Source: CAD feature listing. Evaluate the final solid. Frame: model axes, mm. A direction names the side the tool comes from. Give positions to 0.01 mm unless a question says otherwise; leave off trailing zeros. Loops run counter-clockwise (first coordinate to the right, second up) from the corner with the lowest first, then second, coordinate; pieces in that order, holes last. Notation, with made-up numbers: (-1.75, -39) -> (14.25, -39) arc R24 cw to (14.25, -26) -> close; hole circle Ø10 at (86.25, 67.25). An arc over 180 degrees is marked (long way). Return JSON: item names as keys, results as strings. Group by question number.
(1) Pin query (flat end, axial travel): pin 1 (1.5 mm diameter, centred on x = 1020.5, y = -41.5, fed in from -Z). Return the tip coordinate at first contact, or that it passes through.
(2) Cut plane B-B on y = 353. Return loops of the section in (x, z), then the cut area to 3 significant figures.
(3) Ray query, line 1 (Z direction, x = 579, y = 403.5). Return the intervals inside material, ascending. Write a range as from..to.
(4) Cut plane A-A on x = 301.5. Return loops of the section in (y, z) (3 decimals).
(5) Access query for faces 1 (the face through (1372.587, 32, 101)), 2 (the face through (445, -163, 0)), 3 (the face through (445, 297, 0)). Directions: +Z, -Z, +X, -X, +Y, -Y. A direction counts if a zero-diameter tool reaches every point of the face in a straight line with its end or side. Return the directions, or none.
```python
from build123d import *

# Parameters (mm, degrees)
F0_W     = 1828.8
F0_H     = 914.4
F1_DEPTH = 203.2
F3_R     = 3.175
F4_DEPTH = 1828.8


with BuildPart() as f1:
    # F0 (on Top) → F1 (new body)
    with BuildSketch(Plane.XY):
        with Locations((458.187128, 38.50697)):
            Rectangle(F0_W, F0_H)
    extrude(amount=F1_DEPTH)

    # F3 (on face) → F4 (join)
    with BuildSketch(Plane.YZ.offset(1372.587128)):
        with Locations((89.30697, 0)):
            Circle(F3_R)
    extrude(amount=-F4_DEPTH)


solid = f1.part
```
Answers:
{
 "1": {"pin 1": "z = 0"},
 "2": {"outline": "(-456.21, 0) -> (1372.59, 0) -> (1372.59, 203.2) -> (-456.21, 203.2) -> close", "area": "372,000 mm²"},
 "3": {"line 1": "0..203.2"},
 "4": {"outline": "(-418.693, 0) -> (86.132, 0) arc R3.175 ccw to (92.482, 0) -> (495.707, 0) -> (495.707, 203.2) -> (-418.693, 203.2) -> close"},
 "5": {"face 1": "+Z, -Z, +X, +Y, -Y", "face 2": "-Z, +X, -X, -Y", "face 3": "-Z, +X, -X, +Y"}
}
